Read the model definition and answer for the solid it produces. Units are mm, in the model's axes. Coordinates: 2 decimals unless noted, no trailing zeros. Order: outer loops, then holes, each group sorted by start corner. A loop starts at its lowest first (then second) coordinate and runs counter-clockwise, first axis right, second up.
```python
from build123d import *

# Parameters (mm, degrees)
SKETCH1_W              = 444.5
SKETCH1_H              = 101.6
BOSS_EXTRUDE1_DEPTH    = 6.35
F_10_CLEARANCE_HOLE1_D = 4.9784
F_8_CLEARANCE_HOLE1_D  = 4.3053
SKETCH12_W             = 231.775
SKETCH12_H             = 25.4
CUT_EXTRUDE2_DEPTH     = 229.07021945


with BuildPart() as part:
    # Sketch1 → Boss-Extrude1 (new body)
    with BuildSketch(Plane(origin=(0, 0, 0), x_dir=(0, 0, -1), z_dir=(1, 0, 0))):
        Rectangle(SKETCH1_W, SKETCH1_H)
    extrude(amount=BOSS_EXTRUDE1_DEPTH)

    # #10 Clearance Hole1 (through all)
    with Locations(Plane(origin=(6.35, 0, 0), x_dir=(0, 0, -1), z_dir=(1, 0, 0))):
        with Locations((92.075, 31.75), (92.075, -12.7), (-92.075, 31.75), (-92.075, -12.7)):
            Hole(F_10_CLEARANCE_HOLE1_D / 2)

    # #8 Clearance Hole1 (through all)
    with Locations(Plane(origin=(6.35, 0, 0), x_dir=(0, 0, -1), z_dir=(1, 0, 0))):
        with Locations((-211.328, 35.56), (-211.328, -35.56), (211.328, -35.56), (211.328, 35.56)):
            Hole(F_8_CLEARANCE_HOLE1_D / 2)

    # Sketch12 → Cut-Extrude2 (cut, through all)
    with BuildSketch(Plane(origin=(6.35, 0, 0), x_dir=(0, 0, -1), z_dir=(1, 0, 0))):
        with Locations((0, -38.1)):
            Rectangle(SKETCH12_W, SKETCH12_H)
    extrude(amount=-CUT_EXTRUDE2_DEPTH, mode=Mode.SUBTRACT)


solid = part.part
```
1) Flat-ended cylindrical pins translate along their axes: pin 1 Ø4 at (y, z) = (35.56, 211.328) entering from +X; pin 2 Ø1.9 at (x, z) = (1.5, 33.5) entering from -Y. Find the tip coordinate at first contact, or state that the pin passes through.
A:
pin 1: passes through
pin 2: stops at y = -25.4
2) Straight lines are drawn through the part: line 1 (Z direction, x = 4.25, y = -39); line 2 (Z direction, x = 1.25, y = -34.5); line 3 (Y direction, x = 2, z = -55). For each, find the intervals that lie inside material, in ascending order.
A:
line 1: z = -222.25 to -115.89, 115.89 to 222.25
line 2: z = -222.25 to -213.2, -209.45 to -115.89, 115.89 to 209.45, 213.2 to 222.25
line 3: y = -25.4 to 50.8
3) A cutting plane is placed at A-A, the plane x = 3.5. State how many separate pieces and enclosed holes the cut face has, and give its area (3 significant figures).
A:
separate pieces: 1
enclosed holes: 8
area: 39,100 mm2
4) A cutting plane is placed at B-B, the plane z = 38.5. Determine the outline of the cut face in (x, y), and give its area (3 significant figures).
A:
outline: (0, -25.4) - (6.35, -25.4) - (6.35, 50.8) - (0, 50.8) - close
area: 484 mm2
